The drawing under review shows one solid part. Ordinate dimensions are in mm from its lowest x, y, z. A direction names the side the tool comes from. Round coordinates to 2 decimals unless told otherwise and drop trailing zeros. Write each loop counter-clockwise with the first axis right and the second up, starting at its lowest first coordinate (ties: lowest second). Pieces come first, ordered by that corner, then holes. Notation, with made-up numbers: (83, 85.25) - (142, 85.25) arc R30 ccw to (142, 120.25) - close; hole circle Ø3 at (-29, -20). An arc over 180 degrees is marked (long way). Answer in a Markdown table with one row per item. Add a question column.
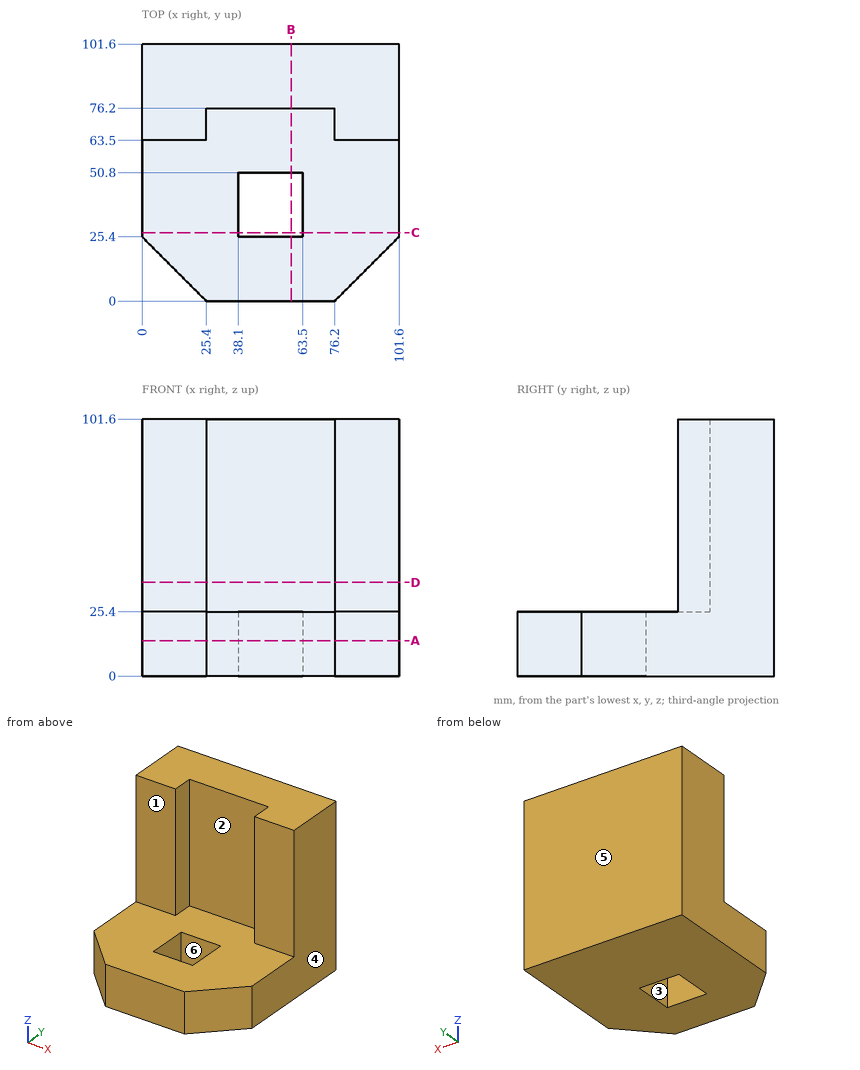
Q1. Add section A-A on z = 14. State the section outline as (x, y) points, then the cut area to 3 significant figures.
Q2. To check wall thickness, follow probe 1 along X at (y, z) = (74.5, 77); probe 2 along X at (y, z) = (36, 23.5); probe 3 along Y at (x, z) = (72, 88). State the ranges of each line that lie inside material, in increasing order.
Q3. Insertion check: pin 1 Ø1 at (x, z) = (30, 51) entering from -Y; pin 2 Ø8 at (y, z) = (18, 14) entering from +X; pin 3 Ø4 at (y, z) = (68.5, 66.5) entering from -X; pin 4 Ø12.5 at (x, z) = (14.5, 45.5) entering from -Y. Each pin has a flat end and moves straight along its axis. Give the tip position at first contact, or say it passes through.
Q4. Add section B-B on x = 59. State the section outline as (y, z) points.
Q5. Add section D-D on z = 37. State the section outline as (x, y) points, then the cut area to 3 significant figures.
Q6. Draft analysis for pull direction Y (two halves, no side actions). For the marked faces 4, 5 and 6, state which applies: released by +Y, released by -Y, zero draft, split by the parting line, or undercut.
Q7. Add section C-C on y = 27. State the section outline as (x, z) points, then the cut area to 3 significant figures.
Q8. Tool access review of the marked faces 1, 2 and 3: name each direction out of +Z, -Z, +X, -X, +Y, -Y from which nothing blocks a thin tool from reaching the whole face with its end or side.
Answer sheet:
| question | item | result |
|---|---|---|
| 1 | outline | (0, 25.4) - (25.4, 0) - (76.2, 0) - (101.6, 25.4) - (101.6, 101.6) - (0, 101.6) - close; hole (38.1, 25.4) - (63.5, 25.4) - (63.5, 50.8) - (38.1, 50.8) - close |
| 1 | area | 9,030 mm² |
| 2 | probe 1 | x = 0 to 25.4, 76.2 to 101.6 |
| 2 | probe 2 | x = 0 to 38.1, 63.5 to 101.6 |
| 2 | probe 3 | y = 76.2 to 101.6 |
| 3 | pin 1 | stops at y = 76.2 |
| 3 | pin 2 | stops at x = 98.2 |
| 3 | pin 3 | stops at x = 0 |
| 3 | pin 4 | stops at y = 63.5 |
| 4 | outline | (0, 0) - (25.4, 0) - (25.4, 25.4) - (0, 25.4) - close; (50.8, 0) - (101.6, 0) - (101.6, 101.6) - (76.2, 101.6) - (76.2, 25.4) - (50.8, 25.4) - close |
| 5 | outline | (0, 63.5) - (25.4, 63.5) - (25.4, 76.2) - (76.2, 76.2) - (76.2, 63.5) - (101.6, 63.5) - (101.6, 101.6) - (0, 101.6) - close |
| 5 | area | 3,230 mm² |
| 6 | face 4 | zero draft |
| 6 | face 5 | released by +Y |
| 6 | face 6 | undercut |
| 7 | outline | (0, 0) - (38.1, 0) - (38.1, 25.4) - (0, 25.4) - close; (63.5, 0) - (101.6, 0) - (101.6, 25.4) - (63.5, 25.4) - close |
| 7 | area | 1,940 mm² |
| 8 | face 1 | +Z, +X, -X, -Y |
| 8 | face 2 | +Z, -Y |
| 8 | face 3 | +Z, -Z |
